Can you work these out from the model? Positions are in its coordinate system, mm. Face numbers are marked on the shaded views. A direction names the side the tool comes from. Give positions to 0.01 mm unless a question says otherwise; leave off trailing zeros. Order: outer loops, then holes, each group sorted by start corner. A loop starts at its lowest first (then second) coordinate and runs counter-clockwise, first axis right, second up. Notation, with made-up numbers: M -18,-37 L 14,-37 A18 cw 14,-28 Z; hole C -15.75,-4.75 d1. An arc over 180 degrees is marked long. One line per question, with ' | ' between items. Start each with the question number.
1) If we section it at A-A, the plane y = 12.5: Please give me the cut outline in (x, z), plus the area to 3 significant figures.
2) If we section it at C-C, the plane z = 49: Please give me the cut outline in (x, y), plus the area to 3 significant figures.
3) If we section it at B-B, the plane x = 0: Please give me the cut outline in (y, z).
4) I'm going to push a flat-ended pin straight in: pin 1 Ø1 at (x, z) = (9.5, -31.5) entering from -Y. Where does the tip first touch, or does it pass through?
5) Please list where these lines run through material, in increasing order: line 1 along Y through (x, z) = (-25, -28); line 2 along Z through (x, y) = (42, 13.6); line 3 along Z through (x, y) = (2, 13.05). Write a range as [from, to].
6) For the marked faces 1 and 2, which set-ups out of +Z, -Z, +X, -X, +Y, -Y let a thin tool reach every point of the face, with its end or its side?
7) If we section it at D-D, the plane z = 24.5: Please give me the cut outline in (x, y).
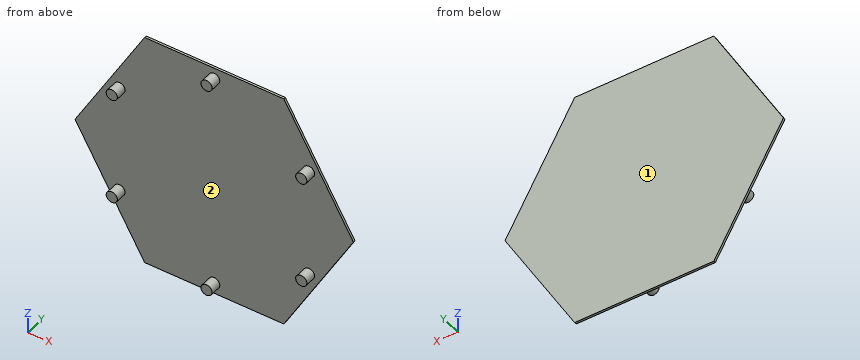
```python
from build123d import *

# Parameters (mm, degrees)
SKETCH1_R             = 2.5
BOSS_EXTRUDE1_DEPTH   = 5
BOSS_EXTRUDE1_2_DEPTH = 5
BOSS_EXTRUDE1_3_DEPTH = 5
BOSS_EXTRUDE1_4_DEPTH = 5
BOSS_EXTRUDE1_5_DEPTH = 5
BOSS_EXTRUDE1_6_DEPTH = 5
BOSS_EXTRUDE2_DEPTH   = 1


with BuildPart() as part:
    # Sketch1 → Boss-Extrude1 (new body)
    with BuildSketch(Plane(origin=(0, 10, 0), x_dir=(1, 0, 0), z_dir=(0, 1, 0))):
        with Locations(Location((0, 49, 0), (0, 0, 270))):
            Circle(SKETCH1_R)
    extrude(amount=BOSS_EXTRUDE1_DEPTH)



with BuildPart() as body_2:
    # Sketch1 → Boss-Extrude1 2 (new body)
    with BuildSketch(Plane(origin=(0, 10, 0), x_dir=(1, 0, 0), z_dir=(0, 1, 0))):
        with Locations(Location((42.435244785, 24.5, 0), (0, 0, 270))):
            Circle(SKETCH1_R)
    extrude(amount=BOSS_EXTRUDE1_2_DEPTH)


with BuildPart() as body_3:
    # Sketch1 → Boss-Extrude1 3 (new body)
    with BuildSketch(Plane(origin=(0, 10, 0), x_dir=(1, 0, 0), z_dir=(0, 1, 0))):
        with Locations(Location((42.435244785, -24.5, 0), (0, 0, 270))):
            Circle(SKETCH1_R)
    extrude(amount=BOSS_EXTRUDE1_3_DEPTH)


with BuildPart() as body_4:
    # Sketch1 → Boss-Extrude1 4 (new body)
    with BuildSketch(Plane(origin=(0, 10, 0), x_dir=(1, 0, 0), z_dir=(0, 1, 0))):
        with Locations(Location((0, -49, 0), (0, 0, 270))):
            Circle(SKETCH1_R)
    extrude(amount=BOSS_EXTRUDE1_4_DEPTH)


with BuildPart() as body_5:
    # Sketch1 → Boss-Extrude1 5 (new body)
    with BuildSketch(Plane(origin=(0, 10, 0), x_dir=(1, 0, 0), z_dir=(0, 1, 0))):
        with Locations(Location((-42.435244785, -24.5, 0), (0, 0, 270))):
            Circle(SKETCH1_R)
    extrude(amount=BOSS_EXTRUDE1_5_DEPTH)


with BuildPart() as body_6:
    # Sketch1 → Boss-Extrude1 6 (new body)
    with BuildSketch(Plane(origin=(0, 10, 0), x_dir=(1, 0, 0), z_dir=(0, 1, 0))):
        with Locations(Location((-42.435244785, 24.5, 0), (0, 0, 270))):
            Circle(SKETCH1_R)
    extrude(amount=BOSS_EXTRUDE1_6_DEPTH)


with BuildPart() as part_1:
    add(part.part)

    add(body_2.part)  # Boss-Extrude2 merges body 2

    add(body_3.part)  # Boss-Extrude2 merges body 3

    add(body_4.part)  # Boss-Extrude2 merges body 4

    add(body_5.part)  # Boss-Extrude2 merges body 5

    add(body_6.part)  # Boss-Extrude2 merges body 6
    # Sketch2 → Boss-Extrude2 (add)
    with BuildSketch(Plane(origin=(0, 15, 0), x_dir=(1, 0, 0), z_dir=(0, 1, 0))):
        Polygon((62.353829072, 0), (31.176914536, 54), (-31.176914536, 54), (-62.353829072, 0), (-31.176914536, -54), (31.176914536, -54), align=None)
    extrude(amount=BOSS_EXTRUDE2_DEPTH)


solid = part_1.part
```
Results found:
1) outline: C -42.44,-24.5 d5; C -42.44,24.5 d5; C 0,-49 d5; C 0,49 d5; C 42.44,-24.5 d5; C 42.44,24.5 d5 | area: 118 mm²
2) outline: M -34.06,15 L -2.5,15 L -2.5,10 L 2.5,10 L 2.5,15 L 34.06,15 L 34.06,16 L -34.06,16 Z | area: 93.1 mm²
3) outline: M 10,-51.5 L 15,-51.5 L 15,-54 L 16,-54 L 16,54 L 15,54 L 15,51.5 L 10,51.5 L 10,46.5 L 15,46.5 L 15,-46.5 L 10,-46.5 Z
4) pin 1: stops at y = 15
5) line 1: y = [15, 16] | line 2: z = [-26.96, -22.04], [22.04, 26.96] | line 3: z = [-50.5, -47.5], [47.5, 50.5]
6) face 1: +Z, -Z, +X, -X, +Y | face 2: -Y
7) outline: M -48.21,15 L -44.94,15 L -44.94,10 L -39.94,10 L -39.94,15 L 39.94,15 L 39.94,10 L 44.94,10 L 44.94,15 L 48.21,15 L 48.21,16 L -48.21,16 Z
